Input: part model. Units: mm. Frame: model coordinates. A direction names the side the tool comes from. Round coordinates to 2 decimals unless told otherwise and drop trailing zeros. Loops run counter-clockwise (first coordinate to the right, second up) from the corner with the lowest first, then second, coordinate; pieces in that order, holes last. Notation, with made-up numbers: (62.25, 24.5) - (115.25, 24.5) arc R7 cw to (115.25, 37.5) - close; hole circle Ø5 at (72.5, 26.5). An arc over 180 degrees is marked (long way). Use CSV: the item, a comma, the result in double quotes. Start each with the question number.
1. Pull-direction query (X, two-part tool) for faces 1 (the flat face through (9, 2, 5)), 2 (the flat face through (12.5, 1.6, 3.8)), 3 (the cylindrical face through (9.87, 0.99, 9.74)); classes: +X half, -X half, draft (parallel to the pull), parting line (faces both ways), or undercut.
2. Cut plane C-C (y = 8.75). Return loops of the section in (x, z), and give its area (3 significant figures).
3. Pin query (flat end, axial travel): P1, Ø3, axis at x = -10, z = 8.75, coming from the +Y side; P2, Ø1.5, axis at x = -3.5, y = 1.5, coming from the +Z side; P3, Ø4, axis at x = -9, y = 6, coming from the +Z side. Return the tip coordinate at first contact, or that it passes through.
4. Cut plane B-B (x = -10). Return loops of the section in (y, z).
5. Material intervals for probe 1 along X at (y, z) = (6, 0.3); probe 2 along Z at (x, y) = (10, 0.7); probe 3 along Y at (x, z) = (-9, 0.65), sorted ascending. Write a range as from..to.
6. Access query for faces 4 (the flat face through (8.335, 0.986, 9.764)), 5 (the flat face through (0.2, 10, 0.5)), 6 (the flat face through (0, 6, 1)). Directions: +Z, -Z, +X, -X, +Y, -Y. A direction counts if a zero-diameter tool reaches every point of the face in a straight line with its end or side. Return the directions, or none.
7. Cut plane A-A (z = 4.75). Return loops of the section in (x, y), and give its area (3 significant figures).
8. Cut plane D-D (x = 4). Return loops of the section in (y, z).
Autodesk Inventor part; units mm, degrees
ref_plane "YZ Plane" through (0, 0, 0) normal (1, 0, 0) x (0, 1, 0)
ref_plane "XZ Plane" through (0, 0, 0) normal (0, 1, 0) x (-1, 0, 0)
ref_plane "XY Plane" through (0, 0, 0) normal (0, 0, 1) x (1, 0, 0)
sketch "スケッチ1" plane through (0, 0, 0) normal (0, 0, 1) x (1, 0, 0)
  line L0 (-12.5, 0) -> (12.5, 0)
  line L1 (12.5, 0) -> (12.5, 10)
  line L2 (12.5, 10) -> (-12.5, 10)
  line L3 (-12.5, 10) -> (-12.5, 0)
  point P0 (0, 0)
  point P1 (0, 0)
  dimension "d0" = 25
  dimension "d1" = 10
extrude "押し出し1" add sketch "スケッチ1" along normal blind 1
sketch "スケッチ2" plane through (-12.5, 0, 0) normal (0, -1, 0) x (1, 0, 0)
  line L0 (12.5, 0) -> (12.5, 16.3622) construction
  circle A0 centre (12.5, 8.75) radius 7.75
  line L1 (0, 1) -> (25, 1) construction
  line L2 (-3.4099, 8.75) -> (28.4099, 8.75) construction
  circle A1 centre (2.5, 8.75) radius 1
  circle A2 centre (22.5, 8.75) radius 1
  line L3 (0, 1) -> (0, 10.75)
  line L4 (0, 1) -> (25, 1)
  line L5 (25, 1) -> (25, 10.75)
  line L6 (0, 10.75) -> (3.5953, 10.75)
  line L7 (3.5953, 10.75) -> (4.75, 8.75)
  line L8 (25, 10.75) -> (21.4047, 10.75)
  line L9 (21.4047, 10.75) -> (20.25, 8.75)
  point P0 (12.5, 1)
  dimension "d4" = 15.5
  dimension "d5" = 2
  dimension "d6" = 20
  dimension "d8" = 2
  dimension "d9" = 60
  dimension "d10" = 60
extrude "押し出し2" add sketch "スケッチ2" against normal blind 2 contours L9 L8 L5 L4 A0 | A0 L4 L3 L6 L7
sketch "スケッチ4" plane through (0, 0, 0) normal (0, 0, -1) x (-1, 0, 0)
  line L0 (18.7059, 6) -> (-18.7059, 6) construction
  line L1 (0, -10.402) -> (0, 10.402) construction
  line L2 (12.5, 0) -> (-12.5, 0) construction
  point P0 (0, 0)
  point P1 (0, 0)
  point P2 (0, 6)
  point P3 (9, 6)
  point P4 (-9, 6)
  dimension "d17" = 18
  dimension "d18" = 6
hole "穴1" at (-9, 6, 0) at (9, 6, 0) direction (0, 0, 1) diameter 3 end through all
equation "\"d10\" = d9"
properties part number "Stepper-D15-S18_Braket"
Established:
1,face 1,"draft"
1,face 2,"+X half"
1,face 3,"undercut"
2,outline,"(-12.5, 0) - (12.5, 0) - (12.5, 1) - (-12.5, 1) - close"
2,area,"25.0 mm2"
3,P1,"stops at y = 2"
3,P2,"stops at z = 2.27"
3,P3,"stops at z = 1"
4,outline,"(0, 0) - (4.88, 0) - (4.88, 1) - (2, 1) - (2, 7.75) - (0, 7.75) - close; (0, 9.75) - (2, 9.75) - (2, 10.75) - (0, 10.75) - close; (7.12, 0) - (10, 0) - (10, 1) - (7.12, 1) - close"
5,probe 1,"x = -12.5..-10.5, -7.5..7.5, 10.5..12.5"
5,probe 2,"z = 0..7.75, 9.75..10.75"
5,probe 3,"y = 0..4.5, 7.5..10"
6,face 4,"+Z, +Y, -Y"
6,face 5,"+Z, -Z, +X, -X, +Y"
6,face 6,"+Z, +X, -X, +Y"
7,outline,"(-12.5, 0) - (-6.64, 0) - (-6.64, 2) - (-12.5, 2) - close; (6.64, 0) - (12.5, 0) - (12.5, 2) - (6.64, 2) - close"
7,area,"23.4 mm2"
8,outline,"(0, 0) - (10, 0) - (10, 1) - (2, 1) - (2, 2.11) - (0, 2.11) - close"
